from build123d import *

# Parameters (mm, degrees)
F0_R     = 26.67
F0_R_2   = 25.7175
F1_DEPTH = 12.7
F0_R_3   = 3.6140603124
F0_R_4   = 2.7324582159
F0_R_5   = 2.6764413385
F0_R_6   = 2.0706768846
F0_R_7   = 2.3053611978
F0_R_8   = 2.0495959377
F2_DEPTH = 2.54
F3_R     = 5.08


# Not quite as in the source:
# - a fillet or chamfer that OpenCascade refuses, or shapes differently, is made with other operations: its cross-section is extruded or revolved along the edge and cut away or added


with BuildPart() as f1:
    # F0 (on Top) → F1 (new body)
    with BuildSketch(Plane.XY):
        Circle(F0_R)
        Circle(F0_R_2, mode=Mode.SUBTRACT)
    extrude(amount=F1_DEPTH)

    # F0 (on Top) → F2 (join)
    with BuildSketch(Plane.XY):
        Circle(F0_R_2)
        with Locations((-0.2498619724, -15.9751214087)):
            Circle(F0_R_3, mode=Mode.SUBTRACT)
        with Locations((-10.1906396449, -8.8177612051)):
            Circle(F0_R_4, mode=Mode.SUBTRACT)
        with Locations((-7.2378846817, 0)):
            Circle(F0_R_5, mode=Mode.SUBTRACT)
        with Locations((0, -6.0694427229)):
            Circle(F0_R_6, mode=Mode.SUBTRACT)
        with Locations((9.885732587, -8.9516246493)):
            Circle(F0_R_4, mode=Mode.SUBTRACT)
        with Locations((5.8176736347, 0)):
            Circle(F0_R_7, mode=Mode.SUBTRACT)
        with Locations((15.1746629134, -0.0083851115)):
            Circle(F0_R_3, mode=Mode.SUBTRACT)
        with Locations((-15.3598431498, 0.1952101447)):
            Circle(F0_R_3, mode=Mode.SUBTRACT)
        with Locations((0, 5.3194356151)):
            Circle(F0_R_8, mode=Mode.SUBTRACT)
        with Locations((-9.527919814, 10.0034438074)):
            Circle(F0_R_4, mode=Mode.SUBTRACT)
        with Locations((0, 13.979755342)):
            Circle(F0_R_3, mode=Mode.SUBTRACT)
        with Locations((8.7631102651, 9.3407258391)):
            Circle(F0_R_4, mode=Mode.SUBTRACT)
    extrude(amount=F2_DEPTH)

    # F3
    f3_edges = [f1.edges().sort_by_distance(p)[0] for p in [
        (-26.67, 0, 0),
    ]]
    fillet(f3_edges, radius=F3_R)

    # F4: fillet of radius 5.08 on 1 edges, made by hand

    # F4_s1 → F4_t2 (revolve, cut)
    with BuildSketch(Plane.XZ):
        with BuildLine():
            ThreePointArc((26.67, 9.7385571506), (26.4260159222, 11.2939831373), (25.7175, 12.7))
            Line((25.7175, 12.7), (26.67, 12.7))
            Line((26.67, 12.7), (26.67, 9.7385571506))
        make_face()
    revolve(axis=Axis((0, 0, 12.7), (0, 0, 1)), mode=Mode.SUBTRACT)


solid = f1.part
Work out the finished part from the listing and answer in its coordinate system (mm). A direction names the side the tool comes from. Round coordinates to 2 decimals unless told otherwise and drop trailing zeros. Write each loop counter-clockwise with the first axis right and the second up, starting at its lowest first coordinate (ties: lowest second). Pieces come first, ordered by that corner, then holes.
1) Straight lines are drawn through the part: line 1 (Y direction, x = 11, z = 2.5); line 2 (Z direction, x = 3, y = -18.5); line 3 (Y direction, x = 14, z = 3.5). For each, find the intervals that lie inside material, in ascending order.
2) A cutting plane is placed at B-B (y = 1). Give the number of separate pieces and of enclosed holes in the cut face, plus the area to 3 significant figures.
3) Given pin 1 Ø9.5 at (x, y) = (15.17, -0.01) entering from +Z; pin 2 Ø2 at (y, z) = (-10.5, 11.5) entering from +X; pin 3 Ø3 at (y, z) = (-19.5, 10) entering from -X, each flat-ended and moving along its own axis, determine where each tip first touches the part or whether it passes through.
4) A cutting plane is placed at A-A (x = 0). Give the vertices of the cut face in (y, z), plus the area to 3 significant figures.
5) A cutting plane is placed at C-C (z = 8). Give the vertices of the cut face in (x, y) (1 decimal), plus the area to 3 significant figures.
6) A tool of negligible diameter and unlimited length cuts with its end or side. For faces 1 (the flat face through (0, 0, 2.54)), 2 (the cylindrical face through (-8.06, 12.31, 1.25)), from which of +Z, -Z, +X, -X, +Y, -Y can it reach the whole face along a straight path? Write none if from no direction.
7) The mould has two halves that part along X. Classify faces 3 (the cylindrical face through (-3.472, 26.443, 7.377)), 4 (the cylindrical face through (-20.41, -15.65, 7.55)), 5 (the flat face through (0, 0, 0)): pulls with the +X half, pulls with the -X half, needs draft (parallel to the pull), parting line crosses it, or undercut.
Completed:
1. line 1: y = -23.52 to -11.45, -6.46 to 7.77, 10.91 to 23.52
1. line 2: z = 0 to 2.54
1. line 3: y = -22.4 to -21.57, 21.57 to 22.4
2. separate pieces: 5
2. enclosed holes: 0
2. area: 83.2 mm2
3. pin 1: stops at z = 2.54
3. pin 2: stops at x = 24.7
3. pin 3: stops at x = -19.67
4. outline: (-26.67, 5.08) arc R5.08 ccw to (-21.59, 0) - (-19.58, 0) - (-19.58, 2.54) - (-25.72, 2.54) - (-25.72, 12.7) arc R5.08 ccw to (-26.67, 9.74) - close; (-12.37, 0) - (-8.14, 0) - (-8.14, 2.54) - (-12.37, 2.54) - close; (-4, 0) - (3.27, 0) - (3.27, 2.54) - (-4, 2.54) - close; (7.37, 0) - (10.37, 0) - (10.37, 2.54) - (7.37, 2.54) - close; (17.59, 0) - (21.59, 0) arc R5.08 ccw to (26.67, 5.08) - (26.67, 9.74) arc R5.08 ccw to (25.72, 12.7) - (25.72, 2.54) - (17.59, 2.54) - close
4. area: 84.4 mm2
5. outline: circle Ø53.3 at (0, 0); hole circle Ø51.4 at (0, 0)
5. area: 157 mm2
6. face 1: +Z
6. face 2: +Z, -Z
7. face 3: parting line crosses it
7. face 4: undercut
7. face 5: needs draft
